Work out the finished part from the listing and answer in its coordinate system (mm). Round coordinates to 2 decimals unless told otherwise and drop trailing zeros. Write each loop counter-clockwise with the first axis right and the second up, starting at its lowest first coordinate (ties: lowest second). Pieces come first, ordered by that corner, then holes. Notation, with made-up numbers: M 50,14.25 L 92,14.25 A11 ccw 92,24.25 Z; hole C 9,18.5 d1. An arc over 180 degrees is marked long. Answer in a Markdown table with one row per item.
```python
from build123d import *

# Parameters (mm, degrees)
BOSS_EXTRUDE1_DEPTH = 20
SKETCH2_W           = 0.5
SKETCH2_H           = 0.5
BOSS_EXTRUDE2_DEPTH = 2
SKETCH3_W           = 0.5
SKETCH3_H           = 0.5
BOSS_EXTRUDE3_DEPTH = 3
FILLET2_R           = 0.1


with BuildPart() as part:
    # Sketch1 → Boss-Extrude1 (new body)
    with BuildSketch(Plane.XY):
        Polygon((0.1, -1.5), (0.1, -1.399682434), (1.901861327, -1.399682434), (1.901861327, -1.5), (2, -1.5), (2, 0), (0, 0), (0, -1.5), align=None)
    extrude(amount=-BOSS_EXTRUDE1_DEPTH)

    # Sketch2 → Boss-Extrude2 (add)
    with BuildSketch(Plane(origin=(0, 0, 0), x_dir=(1, 0, 0), z_dir=(0, 1, 0))):
        with Locations((1, 3.75)):
            Rectangle(SKETCH2_W, SKETCH2_H)
        with Locations((1, 1.25)):
            Rectangle(SKETCH2_W, SKETCH2_H)
        with Locations((1, 6.25)):
            Rectangle(SKETCH2_W, SKETCH2_H)
        with Locations((1, 8.75)):
            Rectangle(SKETCH2_W, SKETCH2_H)
        with Locations((1, 11.25)):
            Rectangle(SKETCH2_W, SKETCH2_H)
        with Locations((1, 13.75)):
            Rectangle(SKETCH2_W, SKETCH2_H)
        with Locations((1, 16.25)):
            Rectangle(SKETCH2_W, SKETCH2_H)
        with Locations((1, 18.75)):
            Rectangle(SKETCH2_W, SKETCH2_H)
    extrude(amount=BOSS_EXTRUDE2_DEPTH)

    # Sketch3 → Boss-Extrude3 (add)
    with BuildSketch(Plane(origin=(0, -1.399682434, 0), x_dir=(-1, 0, 0), z_dir=(0, -1, 0))):
        with Locations((-1, 1.25)):
            Rectangle(SKETCH3_W, SKETCH3_H)
        with Locations((-1, 3.75)):
            Rectangle(SKETCH3_W, SKETCH3_H)
        with Locations((-1, 6.25)):
            Rectangle(SKETCH3_W, SKETCH3_H)
        with Locations((-1, 8.75)):
            Rectangle(SKETCH3_W, SKETCH3_H)
        with Locations((-1, 11.25)):
            Rectangle(SKETCH3_W, SKETCH3_H)
        with Locations((-1, 13.75)):
            Rectangle(SKETCH3_W, SKETCH3_H)
        with Locations((-1, 16.25)):
            Rectangle(SKETCH3_W, SKETCH3_H)
        with Locations((-1, 18.75)):
            Rectangle(SKETCH3_W, SKETCH3_H)
    extrude(amount=BOSS_EXTRUDE3_DEPTH)

    # Fillet2
    fillet2_edges = [part.edges().sort_by_distance(p)[0] for p in [
        (1, 2, -18.5),
        (1.25, 2, -18.75),
        (1, 2, -19),
        (0.75, 2, -18.75),
        (0.75, -4.399682434, -1.25),
        (1, -4.399682434, -1.5),
        (1.25, -4.399682434, -1.25),
        (1, -4.399682434, -1),
        (1, -4.399682434, -3.5),
        (0.75, -4.399682434, -3.75),
        (1, -4.399682434, -4),
        (1.25, -4.399682434, -3.75),
        (1, -4.399682434, -6),
        (0.75, -4.399682434, -6.25),
        (1, -4.399682434, -6.5),
        (1.25, -4.399682434, -6.25),
        (1, -4.399682434, -8.5),
        (0.75, -4.399682434, -8.75),
        (1, -4.399682434, -9),
        (1.25, -4.399682434, -8.75),
        (1, -4.399682434, -11),
        (0.75, -4.399682434, -11.25),
        (1, -4.399682434, -11.5),
        (1.25, -4.399682434, -11.25),
        (1, -4.399682434, -13.5),
        (0.75, -4.399682434, -13.75),
        (1, -4.399682434, -14),
        (1.25, -4.399682434, -13.75),
        (1, -4.399682434, -16),
        (0.75, -4.399682434, -16.25),
        (1, -4.399682434, -16.5),
        (1.25, -4.399682434, -16.25),
        (1, -4.399682434, -18.5),
        (0.75, -4.399682434, -18.75),
        (1, -4.399682434, -19),
        (1.25, -4.399682434, -18.75),
        (1.25, 2, -1.25),
        (1, 2, -1.5),
        (0.75, 2, -1.25),
        (1, 2, -1),
        (1, 2, -3.5),
        (1.25, 2, -3.75),
        (1, 2, -4),
        (0.75, 2, -3.75),
        (1, 2, -6),
        (1.25, 2, -6.25),
        (1, 2, -6.5),
        (0.75, 2, -6.25),
        (1, 2, -8.5),
        (1.25, 2, -8.75),
        (1, 2, -9),
        (0.75, 2, -8.75),
        (1, 2, -11),
        (1.25, 2, -11.25),
        (1, 2, -11.5),
        (0.75, 2, -11.25),
        (1, 2, -13.5),
        (1.25, 2, -13.75),
        (1, 2, -14),
        (0.75, 2, -13.75),
        (1, 2, -16),
        (1.25, 2, -16.25),
        (1, 2, -16.5),
        (0.75, 2, -16.25),
    ]]
    fillet(fillet2_edges, radius=FILLET2_R)


solid = part.part
```
1. Determine the mould class of faces 1 (the flat face through (0, -1, -10)), 2 (the flat face through (1, -1.4, -10)), 3 (the flat face through (1, -1, 0)) for opening direction Z: released by +Z, released by -Z, zero draft, split by the parting line, or undercut.
Calculated:
| item | result |
|---|---|
| face 1 | zero draft |
| face 2 | undercut |
| face 3 | released by +Z |
2. The part is cut by section C-C (x = 0.35). Determine the outline of the cut face in (y, z), plus the area to 3 significant figures.
Calculated:
| item | result |
|---|---|
| outline | M -1.4,-20 L 0,-20 L 0,0 L -1.4,0 Z |
| area | 28.0 mm² |
3. Given pin 1 (0.6 mm diameter, centred on x = 1, y = -2.5, fed in from -Z); pin 2 (0.6 mm diameter, centred on x = 1, y = -3, fed in from +Z), each flat-ended and moving along its own axis, determine where each tip first touches the part or whether it passes through.
Calculated:
| item | result |
|---|---|
| pin 1 | stops at z = -19 |
| pin 2 | stops at z = -1 |
4. The part is cut by section B-B (z = -3). Determine the outline of the cut face in (x, y).
Calculated:
| item | result |
|---|---|
| outline | M 0,-1.5 L 0.1,-1.5 L 0.1,-1.4 L 1.9,-1.4 L 1.9,-1.5 L 2,-1.5 L 2,0 L 0,0 Z |
5. The part is cut by section A-A (y = 1.25). Count the separate pieces of the cut face and the enclosed holes in it, plus the area to 3 significant figures.
Calculated:
| item | result |
|---|---|
| separate pieces | 8 |
| enclosed holes | 0 |
| area | 2.00 mm² |
6. Consider line 1 along Y through (x, z) = (0.35, -16.5); line 2 along X through (y, z) = (0.75, -6.25). Determine where each line is inside the solid, lowest interval first. Write a range as from..to.
Calculated:
| item | result |
|---|---|
| line 1 | y = -1.4..0 |
| line 2 | x = 0.75..1.25 |
